Print and shaded views of the part. All mm, measured from the part's lowest x, y and z. A direction names the side the tool comes from. Round coordinates to 2 decimals unless told otherwise and drop trailing zeros. Write each loop counter-clockwise with the first axis right and the second up, starting at its lowest first coordinate (ties: lowest second). Pieces come first, ordered by that corner, then holes. Notation, with made-up numbers: M -3,2 L 2,2 A32 cw 2,31 Z; hole C 86,89.5 d5. An arc over 180 degrees is marked long. Write item = value, one per line.
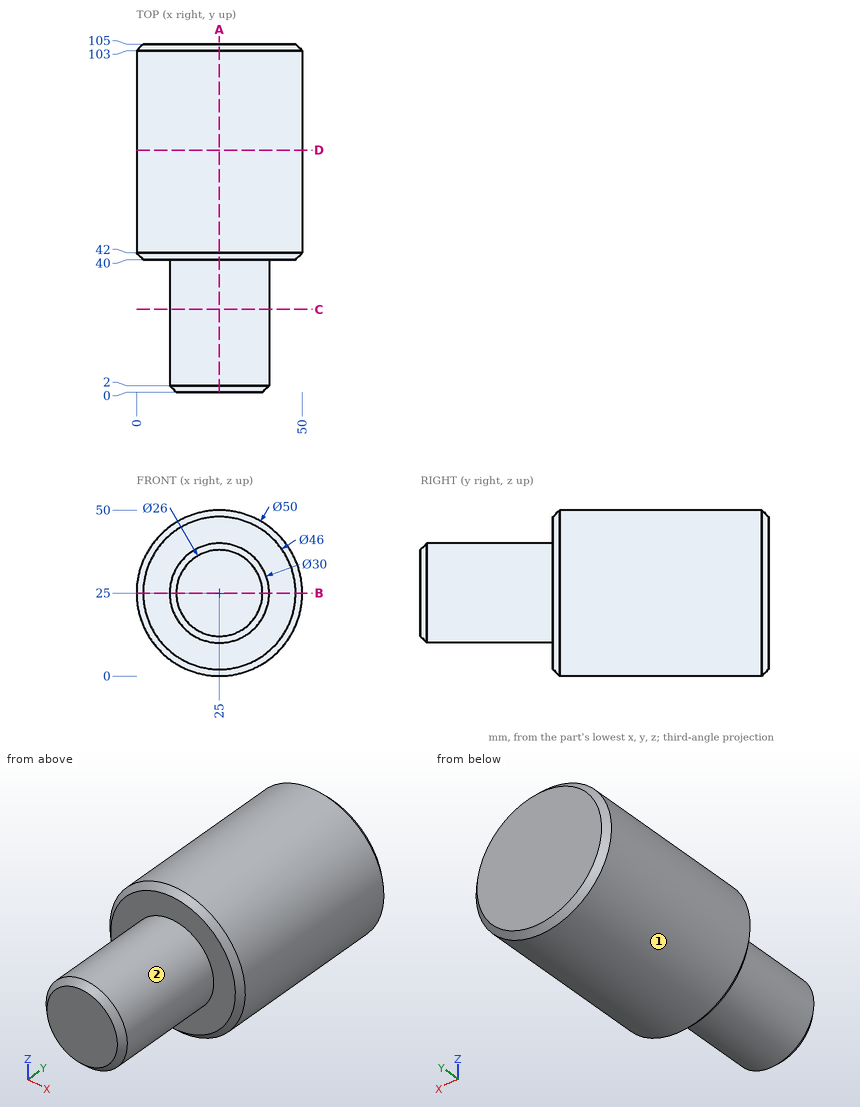
1. Band-saw the part on C-C (y = 25). List the corners of the cut face in (x, z), plus the area to 3 significant figures.
Responses:
outline = C 25,25 d30
area = 707 mm²
2. Band-saw the part on A-A (x = 25). List the corners of the cut face in (y, z).
Responses:
outline = M 0,12 L 2,10 L 40,10 L 40,2 L 42,0 L 103,0 L 105,2 L 105,48 L 103,50 L 42,50 L 40,48 L 40,40 L 2,40 L 0,38 Z
3. Flat gauge pins, fed straight in: pin 1 (10 mm diameter, centred on x = 43.5, y = 74.5, fed in from -Z); pin 2 (8 mm diameter, centred on x = 41.5, z = 44, fed in from -Y); pin 3 (12 mm diameter, centred on x = 35.5, y = 31, fed in from +Z). Where does each tip first touch, or does it go through?
Responses:
pin_1 = 3.96
pin_2 = 40
pin_3 = 39.31
4. Probe probe 1 along Y at (x, z) = (3, 29.5); probe 2 along Z at (x, y) = (45, 56.5); probe 3 along X at (y, z) = (92, 25). List the from-to ranges inside material, lowest first.
Responses:
probe_1 = 40 to 105
probe_2 = 10 to 40
probe_3 = 0 to 50
5. Band-saw the part on D-D (y = 73). List the corners of the cut face in (x, z).
Responses:
outline = C 25,25 d50
6. Tool access for the marked faces 1 and 2: list every direction of +Z, -Z, +X, -X, +Y, -Y with a clear straight run to the whole face (end or side of a thin tool).
Responses:
face_1 = +Y, -Y
face_2 = -Y
7. Band-saw the part on B-B (z = 25). List the corners of the cut face in (x, y), plus the area to 3 significant figures.
Responses:
outline = M 0,42 L 2,40 L 10,40 L 10,2 L 12,0 L 38,0 L 40,2 L 40,40 L 48,40 L 50,42 L 50,103 L 48,105 L 2,105 L 0,103 Z
area = 4,440 mm²
